Here's how the part is built. I have some questions about the finished solid (model axes, mm). A direction names the side the tool comes from. Give positions to 0.01 mm unless a question says otherwise; leave off trailing zeros. Write each loop counter-clockwise with the first axis right and the second up, starting at its lowest first coordinate (ties: lowest second). Pieces come first, ordered by that corner, then holes. Notation, with made-up numbers: (22, 38.5) -> (71, 38.5) arc R11 ccw to (71, 53.5) -> close; hole circle Ø4 at (3.5, -13.5). An arc over 180 degrees is marked (long way). Return JSON: item names as keys, results as strings.
Autodesk Inventor part; units mm, degrees
ref_plane "YZ Plane" through (0, 0, 0) normal (1, 0, 0) x (0, 1, 0)
ref_plane "XZ Plane" through (0, 0, 0) normal (0, 1, 0) x (-1, 0, 0)
ref_plane "XY Plane" through (0, 0, 0) normal (0, 0, 1) x (1, 0, 0)
sketch "Sketch1" plane through (0, 0, 0) normal (0, 1, 0) x (-1, 0, 0)
  circle A0 centre (0, 0) radius 5.1
  circle A1 centre (0, 0) radius 8.95
  dimension "d0" = 10.2
  dimension "d1" = 17.9
extrude "Extrusion1" add sketch "Sketch1" along normal blind 8
chamfer "Chamfer1" distance 2 angle 45 1 edges at (8.95, 8, 0)
sketch "Sketch2" plane through (0, 0, 0) normal (0, -1, 0) x (1, 0, 0)
  circle A0 centre (0, 0) radius 8.95
  circle A1 centre (0, 0) radius 5.1
  circle A2 centre (0, 0) radius 17.5
  dimension "d7" = 35
extrude "Extrusion2" add sketch "Sketch2" along normal blind 6 contours A0 | A2
properties part number "Indre_bøsning_Stempel_stang_3DPrint"
1. Suppose I cut it at D-D, the plane z = -10.5. List the corners of the cut face in (x, y) for me, and give its area (3 significant figures).
Taken from the geometry:
{"outline": "(-14, -6) -> (14, -6) -> (14, 0) -> (-14, 0) -> close", "area": "168 mm²"}
2. Suppose I cut it at B-B, the plane z = 0. List the corners of the cut face in (x, y) for me.
Taken from the geometry:
{"outline": "(-17.5, -6) -> (-5.1, -6) -> (-5.1, 8) -> (-6.95, 8) -> (-8.95, 6) -> (-8.95, 0) -> (-17.5, 0) -> close; (5.1, -6) -> (17.5, -6) -> (17.5, 0) -> (8.95, 0) -> (8.95, 6) -> (6.95, 8) -> (5.1, 8) -> close"}
3. Suppose I cut it at C-C, the plane y = -4.5. List the corners of the cut face in (x, z) for me.
Taken from the geometry:
{"outline": "circle Ø35 at (0, 0); hole circle Ø10.2 at (0, 0)"}
4. Which directions (+Z, -Z, +X, -X, +Y, -Y) give clear straight access to the entire face, cutting with the end or side of a thin tool? Please do faces 1 (the face through (7.1, 2.96, 5.45)), 2 (the face through (4, -6, -4)).
Taken from the geometry:
{"face 1": "+Y", "face 2": "+Z, -Z, +X, -X, -Y"}
5. Suppose I cut it at A-A, the plane x = 0. List the corners of the cut face in (y, z) for me, and give its area (3 significant figures).
Taken from the geometry:
{"outline": "(-6, -17.5) -> (0, -17.5) -> (0, -8.95) -> (6, -8.95) -> (8, -6.95) -> (8, -5.1) -> (-6, -5.1) -> close; (-6, 5.1) -> (8, 5.1) -> (8, 6.95) -> (6, 8.95) -> (0, 8.95) -> (0, 17.5) -> (-6, 17.5) -> close", "area": "206 mm²"}
6. For pin 1 Ø5 at (y, z) = (-3.5, 7) entering from +X; pin 2 Ø1.5 at (y, z) = (6.5, 2) entering from -X; pin 3 Ø5 at (y, z) = (-1.5, -10.5) entering from -X, each with a flat end and sliding along its axis, tell me the tip position at first contact or that it passes through.
Taken from the geometry:
{"pin 1": "stops at x = 16.91", "pin 2": "stops at x = -8.83", "pin 3": "stops at x = -15.56"}
7. If I drill on line 1 (Z direction, x = 0, y = -3.7); line 2 (Y direction, x = -1, z = -13); line 3 (Z direction, x = 2, y = -0.5), over which ranges is the centre line in solid material (lowest first)? Write a range as [from, to].
Taken from the geometry:
{"line 1": "z = [-17.5, -5.1], [5.1, 17.5]", "line 2": "y = [-6, 0]", "line 3": "z = [-17.39, -4.69], [4.69, 17.39]"}
